Here's how the part is built. I have some questions about the finished solid (model axes, mm). Round coordinates to 2 decimals unless told otherwise and drop trailing zeros. Answer as a JSON object with one key per item and string values.
from build123d import *

# Parameters (mm, degrees)
SKICA1_R                                          = 120
SKICA1_R_2                                        = 29
P_IDAT_VYSUNUT_M1_DEPTH                           = 8
KU_ELOV_ZAHLOUBEN_PRO_M8_ROUBY_S_Z_PU_D           = 9
KU_ELOV_ZAHLOUBEN_PRO_M8_ROUBY_S_Z_PU_DEPTH       = 8
KU_ELOV_ZAHLOUBEN_PRO_M8_ROUBY_S_Z_PU_CSINK_D     = 18.92
KU_ELOV_ZAHLOUBEN_PRO_M8_ROUBY_S_Z_PU_CSINK_ANGLE = 90
KU_ELOV_ZAHLOUBEN_PRO_M8_ROUBY_S_Z_PU_TIP         = 2.703872786
ZKOSEN_1_SIZE                                     = 0.5
ZKOSEN_2_SIZE                                     = 0.5
SKICA4_R                                          = 7
ODEBRAT_VYSUNUT_M1_DEPTH                          = 9
KRUHOV_POLE1_COUNT                                = 9
ZKOSEN_3_SIZE                                     = 1
SKICA6_R                                          = 7
ODEBRAT_VYSUNUT_M2_DEPTH                          = 9
KRUHOV_POLE2_COUNT                                = 9


with BuildPart() as part:
    # Skica1 → P_idat vysunut_m1 (new body)
    with BuildSketch(Plane.XY):
        Circle(SKICA1_R)
        Circle(SKICA1_R_2, mode=Mode.SUBTRACT)
    extrude(amount=P_IDAT_VYSUNUT_M1_DEPTH)

    # Ku_elov_ zahlouben_ pro M8 _rouby s z_pu
    with Locations(Plane.XY.offset(8)):
        with Locations((0, 40), (34.641016151, -20), (-34.641016151, -20)):
            CounterSinkHole(KU_ELOV_ZAHLOUBEN_PRO_M8_ROUBY_S_Z_PU_D / 2, KU_ELOV_ZAHLOUBEN_PRO_M8_ROUBY_S_Z_PU_CSINK_D / 2, depth=KU_ELOV_ZAHLOUBEN_PRO_M8_ROUBY_S_Z_PU_DEPTH, counter_sink_angle=KU_ELOV_ZAHLOUBEN_PRO_M8_ROUBY_S_Z_PU_CSINK_ANGLE)
            with Locations((0, 0, -(KU_ELOV_ZAHLOUBEN_PRO_M8_ROUBY_S_Z_PU_DEPTH + KU_ELOV_ZAHLOUBEN_PRO_M8_ROUBY_S_Z_PU_TIP / 2))):  # 118° drill point
                Cone(0, KU_ELOV_ZAHLOUBEN_PRO_M8_ROUBY_S_Z_PU_D / 2, KU_ELOV_ZAHLOUBEN_PRO_M8_ROUBY_S_Z_PU_TIP, mode=Mode.SUBTRACT)

    # Zkosen_1
    zkosen_1_edges = [part.edges().sort_by_distance(p)[0] for p in [
        (-29, 0, 0),
    ]]
    chamfer(zkosen_1_edges, length=ZKOSEN_1_SIZE)

    # Zkosen_2
    zkosen_2_edges = [part.edges().sort_by_distance(p)[0] for p in [
        (-29, 0, 8),
    ]]
    chamfer(zkosen_2_edges, length=ZKOSEN_2_SIZE)

    # Skica4 → Odebrat vysunut_m1 (cut, through all)
    with BuildSketch(Plane.XY.offset(8)):
        with Locations((18.46908774, 50.743401522)):
            Circle(SKICA4_R)
    odebrat_vysunut_m1 = extrude(amount=-ODEBRAT_VYSUNUT_M1_DEPTH, mode=Mode.SUBTRACT)

    # Kruhov_ pole1: Odebrat vysunut_m1 ×9 about axis
    kruhov_pole1_axis = Axis((0, 0, 0), (0, 0, 1))
    for i in range(1, KRUHOV_POLE1_COUNT):
        add(odebrat_vysunut_m1.rotate(kruhov_pole1_axis, i * 360 / KRUHOV_POLE1_COUNT), mode=Mode.SUBTRACT)

    # Zkosen_3
    zkosen_3_edges = [part.edges().sort_by_distance(p)[0] for p in [
        (-120, 0, 0),
        (-120, 0, 8),
    ]]
    chamfer(zkosen_3_edges, length=ZKOSEN_3_SIZE)

    # Skica6 → Odebrat vysunut_m2 (cut, through all)
    with BuildSketch(Plane.XY.offset(8)):
        with Locations((0, 68)):
            Circle(SKICA6_R)
    odebrat_vysunut_m2 = extrude(amount=-ODEBRAT_VYSUNUT_M2_DEPTH, mode=Mode.SUBTRACT)

    # Kruhov_ pole2: Odebrat vysunut_m2 ×9 about axis
    kruhov_pole2_axis = Axis((0, 0, 0), (0, 0, 1))
    for i in range(1, KRUHOV_POLE2_COUNT):
        add(odebrat_vysunut_m2.rotate(kruhov_pole2_axis, i * 360 / KRUHOV_POLE2_COUNT), mode=Mode.SUBTRACT)


solid = part.part
Item 1: I'm going to push flat-ended pins straight in: pin 1 Ø1 at (x, z) = (44, 3) entering from -Y; pin 2 Ø3 at (y, z) = (58, 5.5) entering from +X. Where does each tip first touch, or does it pass through?
Resolved:
{"pin 1": "y = -111.84", "pin 2": "x = 105.87"}
Item 2: I want a section at A-A, the plane x = 0. State how many separate pieces and enclosed holes the cut face has, then the cut area to 3 significant figures.
Resolved:
{"separate pieces": "5", "enclosed holes": "0", "area": "1,130 mm²"}
Item 3: If we mould it in two halves opening along X, with no side actions, what happens to faces 1 (the face through (-64.05, -29.27, 4.06)), 2 (the face through (-119.884, 5.276, 3.958)), 3 (the face through (25, -25, 8))? For each: pulls with the +X half, pulls with the -X half, needs draft (parallel to the pull), parting line crosses it, or undercut.
Resolved:
{"face 1": "undercut", "face 2": "parting line crosses it", "face 3": "needs draft"}
Item 4: Please list where these lines run through material, in increasing order: probe 1 along Y at (x, z) = (0, 2.5); probe 2 along X at (y, z) = (-5, 2.75); probe 3 along X at (y, z) = (-10, 2.5). Write a range as from..to.
Resolved:
{"probe 1": "-120..-61, -47..-29, 29..35.5, 44.5..61, 75..120", "probe 2": "-119.9..-58.64, -47.72..-28.57, 28.57..47.72, 58.64..119.9", "probe 3": "-119.58..-60.15, -46.21..-27.22, 27.22..46.21, 60.15..119.58"}
